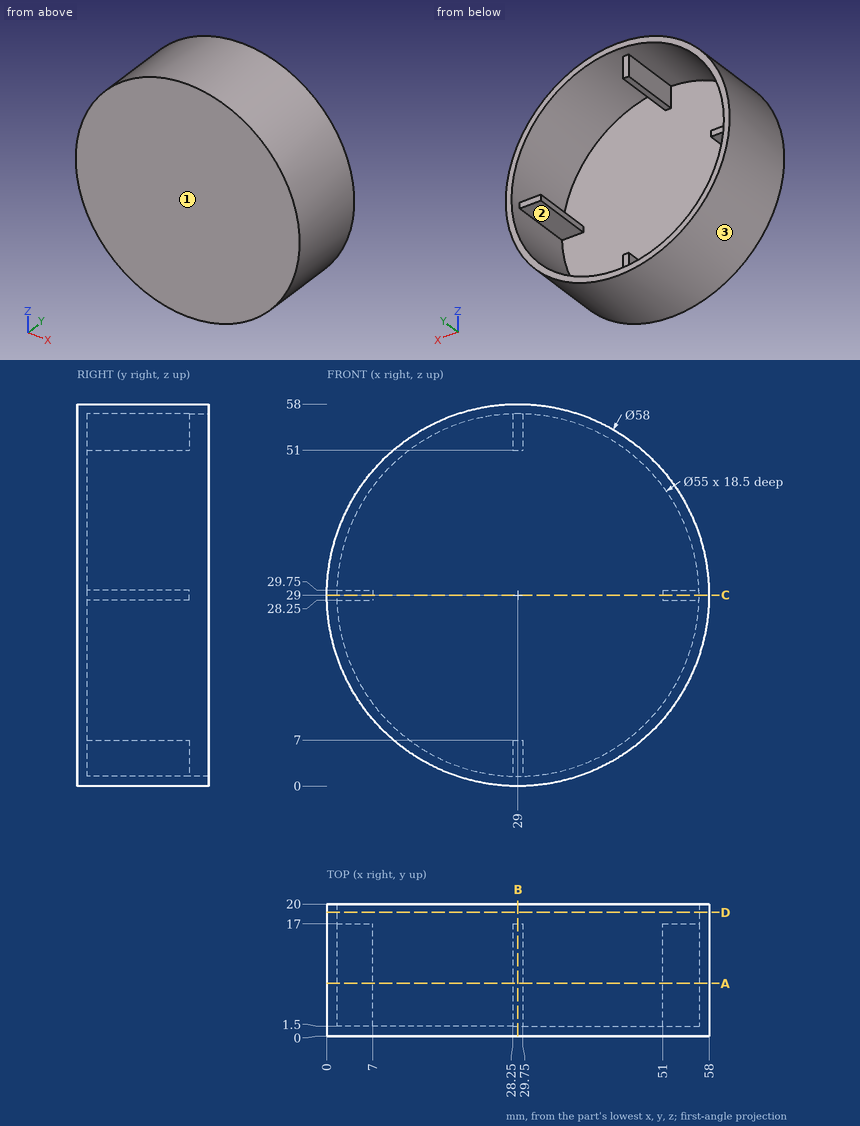
Source: three-view drawing plus pictorial views. Frame: mm from the lowest corner of the part. Give positions to 0.01 mm unless a question says otherwise; leave off trailing zeros. Order: outer loops, then holes, each group sorted by start corner. A loop starts at its lowest first (then second) coordinate and runs counter-clockwise, first axis right, second up. Notation, with made-up numbers: (22.25, 30.5) - (81.25, 30.5) arc R12 ccw to (81.25, 49.5) - close; hole circle Ø3 at (75.5, 27). An arc over 180 degrees is marked (long way). Put each result on its own line as item: value.
Item 1: Section query A-A, the plane y = 8. Return loops of the section in (x, z), then the cut area to 3 significant figures.
Found:
outline: circle Ø58 at (29, 29); hole (1.51, 28.25) arc R27.5 ccw to (28.25, 1.51) - (28.25, 7) - (29.75, 7) - (29.75, 1.51) arc R27.5 ccw to (56.49, 28.25) - (51, 28.25) - (51, 29.75) - (56.49, 29.75) arc R27.5 ccw to (29.75, 56.49) - (29.75, 51) - (28.25, 51) - (28.25, 56.49) arc R27.5 ccw to (1.51, 29.75) - (7, 29.75) - (7, 28.25) - close
area: 299 mm^2
Item 2: Section query C-C, the plane z = 29. Return loops of the section in (x, y).
Found:
outline: (0, 0) - (58, 0) - (58, 20) - (56.5, 20) - (56.5, 17) - (51, 17) - (51, 1.5) - (7, 1.5) - (7, 17) - (1.5, 17) - (1.5, 20) - (0, 20) - close
Item 3: Ray query, L1, parallel to X at y = 16, z = 29; L2, parallel to Y at x = 39, z = 30.5; L3, parallel to Z at x = 6, y = 5.75. Return the intervals inside material, ascending. Write a range as from..to.
Found:
L1: x = 0..7, 51..58
L2: y = 0..1.5
L3: z = 11.34..13.93, 28.25..29.75, 44.07..46.66
Item 4: Contact query for flat-ended pins moving along their axis: pin 1 (6 mm diameter, centred on x = 42.5, y = 16.5, fed in from +Z); pin 2 (3 mm diameter, centred on y = 10.5, z = 28.5, fed in from -X); pin 3 (4 mm diameter, centred on y = 4, z = 49, fed in from -X). Output: stop coordinate, or through.
Found:
pin 1: stops at z = 56.03
pin 2: stops at x = 0
pin 3: stops at x = 6.26
Item 5: Section query D-D, the plane y = 18.75. Return loops of the section in (x, z).
Found:
outline: circle Ø58 at (29, 29); hole circle Ø55 at (29, 29)
Item 6: Draft query along X for the marked faces 1, 2 and 3. Return one class per face: +X half, -X half, draft (parallel to the pull), parting line (faces both ways), or undercut.
Found:
face 1: draft
face 2: undercut
face 3: parting line
Item 7: Section query B-B, the plane x = 29. Return loops of the section in (y, z), then the cut area to 3 significant figures.
Found:
outline: (0, 0) - (20, 0) - (20, 1.5) - (17, 1.5) - (17, 7) - (1.5, 7) - (1.5, 51) - (17, 51) - (17, 56.5) - (20, 56.5) - (20, 58) - (0, 58) - close
area: 313 mm^2
